Work out the finished part from the listing and answer in its coordinate system (mm). Round coordinates to 2 decimals unless told otherwise and drop trailing zeros. Write each loop counter-clockwise with the first axis right and the second up, starting at its lowest first coordinate (ties: lowest second). Pieces come first, ordered by that corner, then holes. Notation, with made-up numbers: (40, -18.5) -> (80, -18.5) arc R28 cw to (80, 5.5) -> close; hole circle Ø10 at (8.5, -8.75). An arc over 180 degrees is marked (long way). One line per question, with ' | ' between items. Start each with the question number.
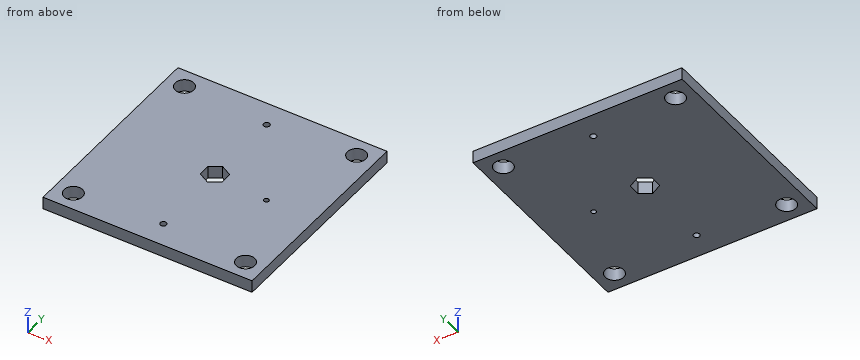
Autodesk Inventor part; units mm, degrees
ref_plane "YZ Plane" through (0, 0, 0) normal (1, 0, 0) x (0, 1, 0)
ref_plane "XZ Plane" through (0, 0, 0) normal (0, 1, 0) x (-1, 0, 0)
ref_plane "XY Plane" through (0, 0, 0) normal (0, 0, 1) x (1, 0, 0)
sketch "Sketch1" plane through (0, 0, 0) normal (0, 0, 1) x (1, 0, 0)
  line L0 (0, 0) -> (170, 0)
  line L1 (170, 0) -> (170, 170)
  line L2 (170, 170) -> (0, 170)
  line L3 (0, 170) -> (0, 0)
  dimension "d0" = 170
  dimension "d1" = 170
extrude "Extrusion1" add sketch "Sketch1" along normal blind 10
sketch "Sketch2" plane through (0, 0, 10) normal (0, 0, 1) x (1, 0, 0)
  line L0 (170, 170) -> (0, 170)
  line L1 (0, 170) -> (0, 155)
  line L2 (0, 170) -> (0, 0)
  line L3 (0, 0) -> (170, 0)
  line L4 (0, 0) -> (0, 15)
  line L5 (0, 15) -> (155, 15)
  line L6 (155, 15) -> (155, 155)
  line L7 (155, 155) -> (15, 155)
  line L8 (15, 155) -> (15, 15)
  line L9 (15, 155) -> (30, 155)
  circle A0 centre (15, 155) radius 7.5
  circle A1 centre (155, 155) radius 7.5
  circle A2 centre (155, 15) radius 7.5
  circle A3 centre (15, 15) radius 7.5
  dimension "d4" = 15
  dimension "d5" = 15
  dimension "d6" = 155
  dimension "d7" = 140
  dimension "d8" = 140
  dimension "d9" = 140
  dimension "d10" = 15
  dimension "d11" = 15
  dimension "d12" = 15
  dimension "d13" = 15
extrude "Extrusion2" cut sketch "Sketch2" against normal blind 10 contours L8 A3 L5 | L5 A3 | L5 A3 L8 | A2 L6 L5 | L5 L6 A2 | A0 L7 L8 | L8 L7 A0 | A1 L7 L6 | L6 L7 A1
sketch "Sketch3" plane through (0, 0, 10) normal (0, 0, 1) x (1, 0, 0)
  line L0 (170, 170) -> (0, 170)
  line L1 (0, 170) -> (85, 170)
  line L2 (85, 170) -> (85, 85)
  line L3 (93.542, 90.1995) -> (93.7739, 80.2022)
  line L4 (93.7739, 80.2022) -> (85.2319, 75.0027)
  line L5 (85.2319, 75.0027) -> (76.458, 79.8005)
  line L6 (76.458, 79.8005) -> (76.2261, 89.7978)
  line L7 (76.2261, 89.7978) -> (84.7681, 94.9973)
  line L8 (84.7681, 94.9973) -> (93.542, 90.1995)
  point P0 (0, 0)
  dimension "d16" = 85
  dimension "d17" = 85
  dimension "d18" = 10
extrude "Extrusion3" cut sketch "Sketch3" against normal blind 10
sketch "Sketch4" plane through (0, 0, 10) normal (0, 0, 1) x (1, 0, 0)
  line L0 (170, 170) -> (0, 170)
  line L1 (0, 170) -> (85, 170)
  line L2 (85, 170) -> (85, 150)
  line L3 (85, 150) -> (85, 20)
  circle A0 centre (85, 150) radius 2.5
  circle A1 centre (85, 20) radius 2.5
  point P0 (0, 0)
  dimension "d21" = 85
  dimension "d22" = 20
  dimension "d23" = 130
  dimension "d24" = 5
  dimension "d25" = 5
extrude "Extrusion4" cut sketch "Sketch4" against normal blind 10
sketch "Sketch5" plane through (0, 0, 10) normal (0, 0, 1) x (1, 0, 0)
  line L0 (170, 0) -> (170, 170)
  line L1 (170, 0) -> (170, 80)
  line L2 (170, 80) -> (130, 80)
  circle A0 centre (130, 80) radius 2
  point P0 (0, 0)
  dimension "d28" = 80
  dimension "d29" = 40
  dimension "d30" = 4
extrude "Extrusion5" cut sketch "Sketch5" against normal blind 10
properties part number "AY"
(1) A cutting plane is placed at A-A, the plane y = 15. Determine the outline of the cut face in (x, z).
(2) A cutting plane is placed at B-B, the plane z = 7. Count the separate pieces of the cut face and the enclosed holes in it, then the cut area to 3 significant figures.
(3) A cutting plane is placed at C-C, the plane y = 84.5. Determine the outline of the cut face in (x, z), then the cut area to 3 significant figures.
(4) Given pin 1 Ø13.5 at (x, y) = (15, 15) entering from -Z; pin 2 Ø6 at (y, z) = (62, 1.5) entering from -X, each flat-ended and moving along its own axis, determine where each tip first touches the part or whether it passes through.
(5) Consider L1, parallel to X at y = 155.5, z = 3; L2, parallel to Y at x = 155, z = 5; L3, parallel to X at y = 20, z = 6.25. Determine where each line is inside the solid, lowest interval first.
Returned:
1) outline: (0, 0) -> (7.5, 0) -> (7.5, 10) -> (0, 10) -> close; (22.5, 0) -> (147.5, 0) -> (147.5, 10) -> (22.5, 10) -> close; (162.5, 0) -> (170, 0) -> (170, 10) -> (162.5, 10) -> close
2) separate pieces: 1 | enclosed holes: 8 | area: 27,900 mm2
3) outline: (0, 0) -> (76.35, 0) -> (76.35, 10) -> (0, 10) -> close; (93.67, 0) -> (170, 0) -> (170, 10) -> (93.67, 10) -> close | area: 1,530 mm2
4) pin 1: through | pin 2: x = 0
5) L1: 0 to 7.52, 22.48 to 147.52, 162.48 to 170 | L2: 0 to 7.5, 22.5 to 147.5, 162.5 to 170 | L3: 0 to 9.41, 20.59 to 82.5, 87.5 to 149.41, 160.59 to 170
